Here's how the part is built. I have some questions about the finished solid (model axes, mm). Face numbers are marked on the shaded views. A direction names the side the tool comes from. Coordinates: 2 decimals unless noted, no trailing zeros. Loops run counter-clockwise (first coordinate to the right, second up) from the corner with the lowest first, then second, coordinate; pieces in that order, holes last. Notation, with made-up numbers: (30, -32) -> (78, -32) arc R33 ccw to (78, -4) -> close; hole circle Ø11 at (64.25, 14). An arc over 180 degrees is marked (long way). Answer as a JSON object with one key per item and string values. Group by question number.
Q1. I want a section at B-B on y = -28. Count the separate pieces of the cut face and the enclosed holes in it, then the cut area to 3 significant figures.
Q2. I want a section at A-A on y = -10. Write out the boundary of the cut face in (x, z).
Q3. I'm going to push flat-ended pins straight in: pin 1 (5.5 mm diameter, centred on x = -6.5, y = -9.5, fed in from -Z); pin 2 (1.1 mm diameter, centred on x = -7.5, z = -0.5, fed in from -Y); pin 3 (1.7 mm diameter, centred on y = -29.5, z = 0.5, fed in from -X). Where does each tip first touch, or does it pass through?
Q4. On a 3-axis mill with a long thin cutter (end or side, diameter ignored), from which of +Z, -Z, +X, -X, +Y, -Y can I reach the whole of each face in a straight line? I mean the marked faces 1, 2 and 3. Say none if no direction works.
Q5. Thinking about a two-plate mould opening in Y: for the marked faces 4, 5 and 6, which applies, released by +Y, released by -Y, zero draft, split by the parting line, or undercut?
Q6. I need wall thicknesses on line 1 (Y direction, x = 0, z = -2); line 2 (Y direction, x = 1.75, z = 3); line 3 (X direction, y = -35.1, z = 1.9). Which ranges of each line are inside material? Lowest first, please.
Q7. I want a section at C-C on z = -3.75. Write out the boundary of the cut face in (x, y).
```python
from build123d import *

# Parameters (mm, degrees)
F1_DEPTH       = 5
F3_DEPTH       = 5
F5_D           = 3.3
F5_DEPTH       = 26
F5_CBORE_D     = 6.5
F5_CBORE_DEPTH = 1
F5_TIP         = 0.9914200214
F7_DEPTH       = 3
F9_DEPTH       = 1.5
F10_D          = 5.5
F10_DEPTH      = 26
F10_TIP        = 1.6523667023
F11_SIZE       = 0.5
F13_R          = 5
F14_SIZE       = 0.5


with BuildPart() as f1:
    # F0 (on Top) → F1 (new body)
    with BuildSketch(Plane.XY):
        with BuildLine():
            Line((10, 0), (-10, 0))
            Line((-10, 0), (-10, -35.1))
            ThreePointArc((-10, -35.1), (-7.0710678119, -42.1710678119), (0, -45.1))
            ThreePointArc((0, -45.1), (7.0710678119, -42.1710678119), (10, -35.1))
            Line((10, -35.1), (10, -23))
            Line((10, -23), (4.1, -23))
            Line((4.1, -23), (4.1, -32.0668498224))
            ThreePointArc((4.1, -32.0668498224), (-3.4177556675, -38.8853594542), (2.6, -30.7125178063))
            Line((2.6, -30.7125178063), (2.6, -22))
            Line((2.6, -22), (10, -22))
            Line((10, -22), (10, 0))
        make_face()
    extrude(amount=F1_DEPTH)

    # F2 (on face) → F3 (join)
    with BuildSketch(Plane(origin=(0, 0, 0), x_dir=(1, 0, 0), z_dir=(0, 0, -1))):
        with BuildLine():
            Line((-10, 35.1), (-10, 20))
            Line((-10, 20), (10, 20))
            Line((10, 20), (10, 22))
            Line((10, 22), (2.6, 22))
            Line((2.6, 22), (2.6, 30.7125178063))
            ThreePointArc((2.6, 30.7125178063), (-3.4177556675, 38.8853594542), (4.1, 32.0668498224))
            Line((4.1, 32.0668498224), (4.1, 23))
            Line((4.1, 23), (10, 23))
            Line((10, 23), (10, 35.1))
            ThreePointArc((10, 35.1), (0, 45.1), (-10, 35.1))
        make_face()
    extrude(amount=F3_DEPTH)

    # F5
    with Locations(Plane.YZ.offset(10)):
        with Locations((-28.2125178063, 0)):
            CounterBoreHole(F5_D / 2, F5_CBORE_D / 2, F5_CBORE_DEPTH, depth=F5_DEPTH)
            with Locations((0, 0, -(F5_DEPTH + F5_TIP / 2))):  # 118° drill point
                Cone(0, F5_D / 2, F5_TIP, mode=Mode.SUBTRACT)

    # F6 (on face) → F7 (cut)
    with BuildSketch(Plane(origin=(-10, 0, 0), x_dir=(0, -1, 0), z_dir=(-1, 0, 0))):
        with BuildLine():
            Line((24.9216212719, 0), (26.5670695391, -2.85))
            Line((26.5670695391, -2.85), (29.8579660735, -2.85))
            Line((29.8579660735, -2.85), (31.5034143407, 0))
            Line((31.5034143407, 0), (29.8625178063, 0))
            ThreePointArc((29.8625178063, 0), (28.2125178063, -1.65), (26.5625178063, 0))
            Line((26.5625178063, 0), (24.9216212719, 0))
        make_face()
        with BuildLine():
            Line((26.5670695391, 2.85), (24.9216212719, 0))
            Line((24.9216212719, 0), (26.5625178063, 0))
            ThreePointArc((26.5625178063, 0), (28.2125178063, 1.65), (29.8625178063, 0))
            Line((29.8625178063, 0), (31.5034143407, 0))
            Line((31.5034143407, 0), (29.8579660735, 2.85))
            Line((29.8579660735, 2.85), (26.5670695391, 2.85))
        make_face()
    extrude(amount=-F7_DEPTH, mode=Mode.SUBTRACT)

    # F8 (on face) → F9 (join)
    with BuildSketch(Plane(origin=(0, 0, 0), x_dir=(1, 0, 0), z_dir=(0, 0, -1))):
        with BuildLine():
            ThreePointArc((-4.6097722286, 7), (-5.5, 10), (-4.6097722286, 13))
            Line((-4.6097722286, 13), (-10, 13))
            Line((-10, 13), (-10, 7))
            Line((-10, 7), (-4.6097722286, 7))
        make_face()
        with BuildLine():
            Line((10, 7), (10, 13))
            Line((10, 13), (4.6097722286, 13))
            ThreePointArc((4.6097722286, 13), (5.5, 10), (4.6097722286, 7))
            Line((4.6097722286, 7), (10, 7))
        make_face()
    extrude(amount=F9_DEPTH)

    # F10
    with Locations(Plane(origin=(0, 0, 0), x_dir=(1, 0, 0), z_dir=(0, 0, -1))):
        with Locations((0, 10)):
            Hole(F10_D / 2, depth=F10_DEPTH)
            with Locations((0, 0, -(F10_DEPTH + F10_TIP / 2))):  # 118° drill point
                Cone(0, F10_D / 2, F10_TIP, mode=Mode.SUBTRACT)

    # F11
    f11_edges = [f1.edges().sort_by_distance(p)[0] for p in [
        (-7.304886, -7, -1.5),
        (-7.304886, -13, -1.5),
        (7.304886, -13, -1.5),
        (7.304886, -7, -1.5),
    ]]
    chamfer(f11_edges, length=F11_SIZE)

    # F13
    f13_edges = [f1.edges().sort_by_distance(p)[0] for p in [
        (10, 0, 2.5),
        (-10, 0, 2.5),
    ]]
    fillet(f13_edges, radius=F13_R)

    # F14
    f14_edges = [f1.edges().sort_by_distance(p)[0] for p in [
        (10, -13.5, 5),
        (8.535534, -1.464466, 5),
        (6.3, -22, 5),
        (0, 0, 5),
        (2.6, -26.356259, 5),
        (-8.535534, -1.464466, 5),
        (-3.417756, -38.885359, 5),
        (-10, -20.05, 5),
        (4.1, -27.533425, 5),
        (0, -45.1, 5),
        (7.05, -23, 5),
        (10, -29.05, 5),
        (-2.75, -10, 5),
        (0, -45.1, -5),
        (-10, -27.55, -5),
        (0, -20, -5),
        (10, -21, -5),
        (6.3, -22, -5),
        (2.6, -26.356259, -5),
        (-3.417756, -38.885359, -5),
        (4.1, -27.533425, -5),
        (7.05, -23, -5),
        (10, -29.05, -5),
    ]]
    chamfer(f14_edges, length=F14_SIZE)


solid = f1.part
```
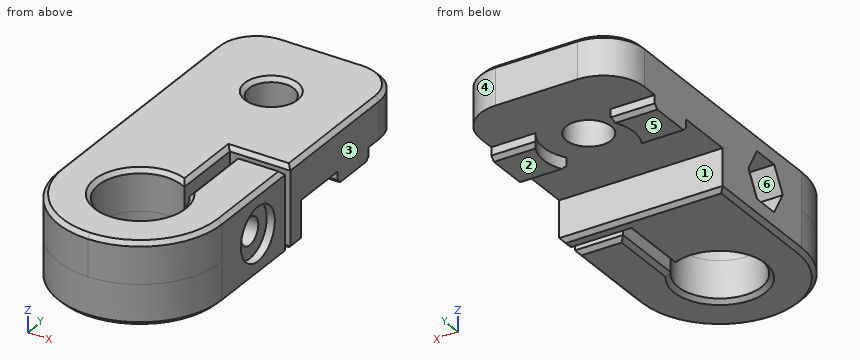
Result set:
{
 "1": {"separate pieces": "4", "enclosed holes": "0", "area": "113 mm²"},
 "2": {"outline": "(-10, -1.5) -> (-5.5, -1.5) -> (-5.5, 0) -> (-2.75, 0) -> (-2.75, 4.5) -> (-3.25, 5) -> (-9.5, 5) -> (-10, 4.5) -> close; (2.75, 0) -> (5.5, 0) -> (5.5, -1.5) -> (10, -1.5) -> (10, 4.5) -> (9.5, 5) -> (3.25, 5) -> (2.75, 4.5) -> close"},
 "3": {"pin 1": "stops at z = -1.5", "pin 2": "stops at y = -42.29", "pin 3": "stops at x = -7"},
 "4": {"face 1": "-Z, +X, -X", "face 2": "-Z, +X, -X, +Y", "face 3": "+Z, -Z, +X, +Y, -Y"},
 "5": {"face 4": "released by +Y", "face 5": "zero draft", "face 6": "undercut"},
 "6": {"line 1": "y = -45.1 to -40.2, -30 to -20", "line 2": "y = -44.95 to -39.89, -30.31 to -12.12, -7.88 to 0", "line 3": "x = -10 to -5.1, 5.1 to 10"},
 "7": {"outline": "(-10, -35.1) arc R10 ccw to (10, -35.1) -> (10, -23) -> (4.1, -23) -> (4.1, -32.07) arc R5.1 cw (long way) to (2.6, -30.71) -> (2.6, -22) -> (10, -22) -> (10, -20) -> (-10, -20) -> close"}
}
